CAD build for the part. Positions are in the model's coordinates, mm. A direction names the side the tool comes from. Round coordinates to 2 decimals unless told otherwise and drop trailing zeros. Order: outer loops, then holes, each group sorted by start corner. A loop starts at its lowest first (then second) coordinate and runs counter-clockwise, first axis right, second up. Notation, with made-up numbers: M -17,59.25 L 31,59.25 A37 cw 31,97.25 Z; hole C 44,-35 d3. An arc over 180 degrees is marked long. Answer as CSV lines item,"result". Start each with the question number.
```python
from build123d import *

# Parameters (mm, degrees)
F0_W     = 30
F0_H     = 60
F1_DEPTH = 10
F2_R     = 3.9
F3_DEPTH = 8
F4_SIZE  = 0.75


with BuildPart() as f1:
    # F0 (on Top) → F1 (new body)
    with BuildSketch(Plane.XY):
        Rectangle(F0_W, F0_H)
    extrude(amount=F1_DEPTH)

    # F2 (on face) → F3 (cut)
    with BuildSketch(Plane.XY.offset(10)):
        with BuildLine():
            ThreePointArc((-15, 12.309584), (-2.102084, 5.752778), (7, 17))
            ThreePointArc((7, 17), (-2.102084, 28.247222), (-15, 21.690416))
            Line((-15, 21.690416), (-15, 12.309584))
        make_face()
        with Locations((-4.5, 17)):
            Circle(F2_R, mode=Mode.SUBTRACT)
        with BuildLine():
            ThreePointArc((7, -17), (-2.102084, -5.752778), (-15, -12.309584))
            Line((-15, -12.309584), (-15, -21.690416))
            ThreePointArc((-15, -21.690416), (-2.102084, -28.247222), (7, -17))
        make_face()
        with Locations((-4.5, -17)):
            Circle(F2_R, mode=Mode.SUBTRACT)
    extrude(amount=-F3_DEPTH, mode=Mode.SUBTRACT)

    # F4
    f4_edges = [f1.edges().sort_by_distance(p)[0] for p in [
        (-8.4, 17, 2),
        (-8.4, -17, 2),
    ]]
    chamfer(f4_edges, length=F4_SIZE)


solid = f1.part
```
Q1. Band-saw the part on C-C, the plane y = 6.5. Write the cut outline in (x, z), then the cut area to 3 significant figures.
Q2. Tool access for faces 1 (the flat face through (1, -17, 2)), 2 (the flat face through (-5, 17, 10)): list every direction of +Z, -Z, +X, -X, +Y, -Y with a clear straight run to the whole face (end or side of a thin tool).
Q3. Band-saw the part on A-A, the plane x = -4.5. Write the cut outline in (y, z), then the cut area to 3 significant figures.
Q4. Band-saw the part on B-B, the plane z = 4.5. Write the cut outline in (x, y), then the cut area to 3 significant figures.
Q5. Band-saw the part on D-D, the plane x = 4. Write the cut outline in (y, z), then the cut area to 3 significant figures.
Q6. Mould opens along Y. For faces 3 (the flat face through (0, 0, 0)), 4 (the flat face through (1, 17, 2)), 5 (the flat face through (0, -30, 5)) say: +Y half, -Y half, draft (parallel to the pull), parting line (faces both ways), or undercut.
Q7. Drop a flat-ended pin along its axis: P1, Ø8, axis at x = -3, y = 0.5, coming from the -Z side. Give the stop position or say it passes through.
Q8. Probe line 1 along Y through (x, z) = (-10.5, 4.25); line 2 along Y through (x, z) = (5.5, 6.5); line 3 along Z through (x, y) = (-5.75, -24). List the from-to ranges inside material, lowest first. Write a range as from..to.
Answer:
1,outline,"M -15,0 L 15,0 L 15,10 L 0.19,10 L 0.19,2 L -9.19,2 L -9.19,10 L -15,10 Z"
1,area,"225 mm^2"
2,face 1,"+Z"
2,face 2,"+Z, +X, -X, +Y, -Y"
3,outline,"M -30,0 L 30,0 L 30,10 L 28.5,10 L 28.5,2 L 21.65,2 L 20.9,2.75 L 20.9,10 L 13.1,10 L 13.1,2.75 L 12.35,2 L 5.5,2 L 5.5,10 L -5.5,10 L -5.5,2 L -12.35,2 L -13.1,2.75 L -13.1,10 L -20.9,10 L -20.9,2.75 L -21.65,2 L -28.5,2 L -28.5,10 L -30,10 Z"
3,area,"358 mm^2"
4,outline,"M -15,-30 L 15,-30 L 15,30 L -15,30 L -15,21.69 A11.5 cw long -15,12.31 L -15,-12.31 A11.5 cw long -15,-21.69 Z; C -4.5,-17 d7.8; C -4.5,17 d7.8"
4,area,"1,080 mm^2"
5,outline,"M -30,0 L 30,0 L 30,10 L 24.75,10 L 24.75,2 L 9.25,2 L 9.25,10 L -9.25,10 L -9.25,2 L -24.75,2 L -24.75,10 L -30,10 Z"
5,area,"352 mm^2"
6,face 3,"draft"
6,face 4,"undercut"
6,face 5,"-Y half"
7,P1,"stops at z = 0"
8,line 1,"y = -30..-26.81, -7.19..7.19, 26.81..30"
8,line 2,"y = -30..-22.68, -11.32..11.32, 22.68..30"
8,line 3,"z = 0..2"
